Here's how the part is built. I have some questions about the finished solid (model axes, mm). Coordinates: 2 decimals unless noted, no trailing zeros. Write each loop counter-clockwise with the first axis right and the second up, starting at its lowest first coordinate (ties: lowest second). Pieces come first, ordered by that corner, then holes.
```python
from build123d import *

# Parameters (mm, degrees)
SKETCH_1_W          = 40.35
SKETCH_1_H          = 70.4
EXTRUDE_1_DEPTH     = 4
SKETCH_2_W          = 2
SKETCH_2_H          = 6.05
SKETCH_2_H_2        = 6.35
SKETCH_2_W_2        = 10
SKETCH_2_H_3        = 25
CUT_EXTRUDE_3_DEPTH = 82.242122695
SKETCH_4_W          = 3
SKETCH_4_H          = 4
CUT_EXTRUDE_4_DEPTH = 82.242122695
SKETCH_5_W          = 6.45
SKETCH_5_H          = 4
EXTRUDE_2_DEPTH     = 5
CHAMFER_1_SIZE      = 5
SKETCH_6_W          = 6.1
SKETCH_6_H          = 4
EXTRUDE_3_DEPTH     = 2


with BuildPart() as part:
    # ｽｹｯﾁ1 → ﾎﾞｽ - 押し出し1 (new body)
    with BuildSketch(Plane(origin=(0, 0, 0), x_dir=(1, 0, 0), z_dir=(0, 1, 0))):
        with Locations((20.175, 35.2)):
            Rectangle(SKETCH_1_W, SKETCH_1_H)
    extrude(amount=EXTRUDE_1_DEPTH)

    # ｽｹｯﾁ2 → ｶｯﾄ - 押し出し3 (cut, through all)
    with BuildSketch(Plane(origin=(0, 4, 0), x_dir=(1, 0, 0), z_dir=(0, 1, 0))):
        with Locations((1, 13.475)):
            Rectangle(SKETCH_2_W, SKETCH_2_H)
        with Locations((39.35, 13.475)):
            Rectangle(SKETCH_2_W, SKETCH_2_H)
        with Locations((1, 62.225)):
            Rectangle(SKETCH_2_W, SKETCH_2_H_2)
        with Locations((39.35, 62.225)):
            Rectangle(SKETCH_2_W, SKETCH_2_H_2)
        with Locations((20.175, 57.9)):
            Rectangle(SKETCH_2_W_2, SKETCH_2_H_3)
    extrude(amount=-CUT_EXTRUDE_3_DEPTH, mode=Mode.SUBTRACT)

    # ｽｹｯﾁ4 → ｶｯﾄ - 押し出し4 (cut, through all)
    with BuildSketch(Plane(origin=(0, 4, 0), x_dir=(1, 0, 0), z_dir=(0, 1, 0))):
        with Locations((12.675, 67.4)):
            Rectangle(SKETCH_4_W, SKETCH_4_H)
        with Locations((12.675, 59.4)):
            Rectangle(SKETCH_4_W, SKETCH_4_H)
        with Locations((12.675, 51.4)):
            Rectangle(SKETCH_4_W, SKETCH_4_H)
        with Locations((27.675, 67.4)):
            Rectangle(SKETCH_4_W, SKETCH_4_H)
        with Locations((27.675, 59.4)):
            Rectangle(SKETCH_4_W, SKETCH_4_H)
        with Locations((27.675, 51.4)):
            Rectangle(SKETCH_4_W, SKETCH_4_H)
    extrude(amount=-CUT_EXTRUDE_4_DEPTH, mode=Mode.SUBTRACT)

    # ｽｹｯﾁ5 → ﾎﾞｽ - 押し出し2 (add)
    with BuildSketch(Plane(origin=(0, 0, -70.4), x_dir=(-1, 0, 0), z_dir=(0, 0, -1))):
        with Locations((-34.125, 2)):
            Rectangle(SKETCH_5_W, SKETCH_5_H)
        with Locations((-6.225, 2)):
            Rectangle(SKETCH_5_W, SKETCH_5_H)
    extrude(amount=EXTRUDE_2_DEPTH)

    # 面取り1
    chamfer_1_edges = [part.edges().sort_by_distance(p)[0] for p in [
        (3, 2, -75.4),
        (37.35, 2, -75.4),
    ]]
    chamfer(chamfer_1_edges, length=CHAMFER_1_SIZE - 0.0001)  # a hair under: the kernel refuses the full size

    # ｽｹｯﾁ6 → ﾎﾞｽ - 押し出し3 (add)
    with BuildSketch(Plane.XY):
        with Locations((6.05, 2)):
            Rectangle(SKETCH_6_W, SKETCH_6_H)
        with Locations((34.3, 2)):
            Rectangle(SKETCH_6_W, SKETCH_6_H)
    extrude(amount=EXTRUDE_3_DEPTH)


solid = part.part
```
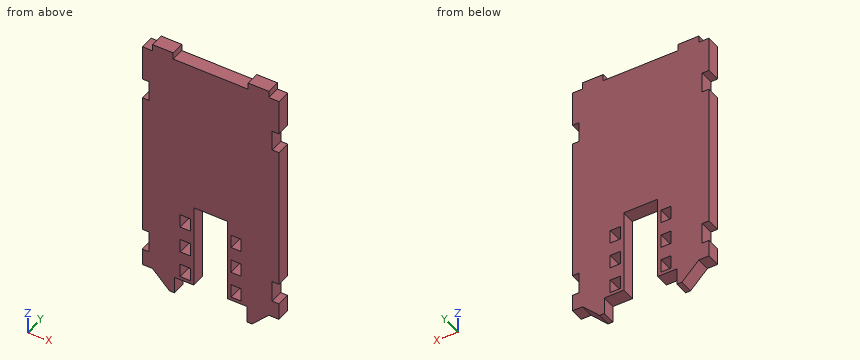
1) Imagine slicing it at B-B on z = -55. Please give me the cut outline in (x, y) (3 decimals), then the cut area to 3 significant figures.
Values follow:
outline: (0, 0) - (15.175, 0) - (15.175, 4) - (0, 4) - close; (25.175, 0) - (40.35, 0) - (40.35, 4) - (25.175, 4) - close
area: 121 mm2
2) Imagine slicing it at C-C on y = 1. Count the separate pieces of the cut face and the enclosed holes in it, then the cut area to 3 significant figures.
Values follow:
separate pieces: 1
enclosed holes: 6
area: 2,530 mm2
3) I need wall thicknesses on probe 1 along Z at (x, y) = (27, 0.2); probe 2 along X at (y, z) = (0.6, -66) (3 decimals); probe 3 along X at (y, z) = (0.35, -59.5) (3 decimals). Which ranges of each line are inside material? Lowest first, please.
Values follow:
probe 1: z = -70.4 to -69.4, -65.4 to -61.4, -57.4 to -53.4, -49.4 to 0
probe 2: x = 0 to 11.175, 14.175 to 15.175, 25.175 to 26.175, 29.175 to 40.35
probe 3: x = 2 to 11.175, 14.175 to 15.175, 25.175 to 26.175, 29.175 to 38.35
4) Will these pins go through, and if not, where does the flat tip stop? pin 1 (0.6 mm diameter, centred on y = 3, z = 0.5, fed in from -X); pin 2 (1.5 mm diameter, centred on x = 27.5, y = 2, fed in from -Z); pin 3 (1.2 mm diameter, centred on y = 2, z = -62, fed in from +X).
Values follow:
pin 1: stops at x = 3
pin 2: stops at z = -70.4
pin 3: stops at x = 38.35
5) Imagine slicing it at D-D on x = 21.5. Please give me the cut outline in (y, z).
Values follow:
outline: (0, -45.4) - (4, -45.4) - (4, 0) - (0, 0) - close
6) Imagine slicing it at A-A on z = -68. Please give me the cut outline in (x, y) (3 decimals).
Values follow:
outline: (0, 0) - (11.175, 0) - (11.175, 4) - (0, 4) - close; (14.175, 0) - (15.175, 0) - (15.175, 4) - (14.175, 4) - close; (25.175, 0) - (26.175, 0) - (26.175, 4) - (25.175, 4) - close; (29.175, 0) - (40.35, 0) - (40.35, 4) - (29.175, 4) - close
